Here's the drawing with two shaded views (mm, measured from the low corner). I have some questions. A direction names the side the tool comes from. Give positions to 0.01 mm unless a question says otherwise; leave off trailing zeros. Order: outer loops, then holes, each group sorted by start corner. A loop starts at its lowest first (then second) coordinate and runs counter-clockwise, first axis right, second up. Notation, with made-up numbers: M 6.5,46.25 L 46.5,46.25 A28 cw 46.5,72.25 Z; hole C -6,-3 d7. An arc over 180 degrees is marked long. Use a Markdown table: item, result. Add a question column.
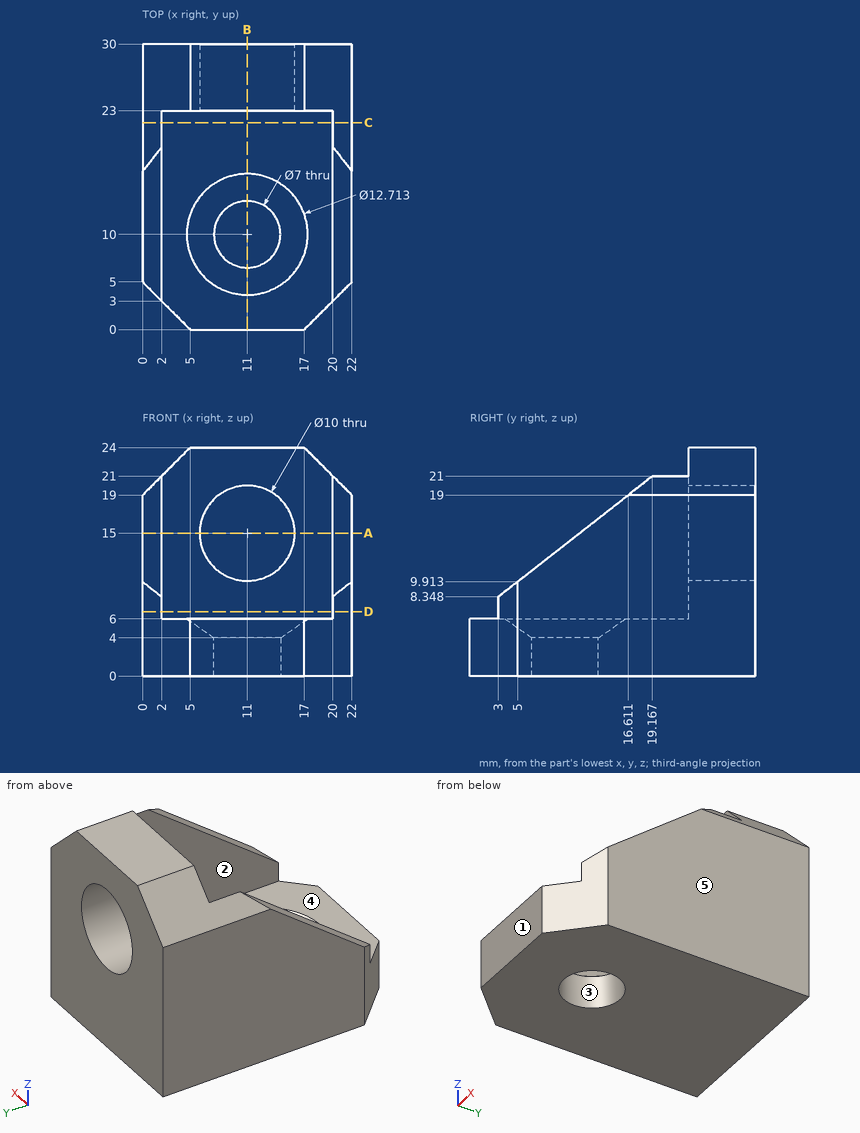
1. If we section it at A-A, the plane z = 15: List the corners of the cut face in (x, y) for me.
2. On a 3-axis mill with a long thin cutter (end or side, diameter ignored), from which of +Z, -Z, +X, -X, +Y, -Y can I reach the whole of each face in a straight line? I mean the marked faces 4 and 5. Say none if no direction works.
3. I need wall thicknesses on L1, parallel to X at y = 13.75, z = 14.25; L2, parallel to Y at x = 11, z = 1.2; L3, parallel to Z at x = 11, y = 28.25. Which ranges of each line are inside material? Lowest first, please. Write a range as [from, to].
4. If we section it at C-C, the plane y = 21.75: List the corners of the cut face in (x, z) for me, then the cut area to 3 significant figures.
5. If we section it at D-D, the plane z = 6.75: List the corners of the cut face in (x, y) for me, then the cut area to 3 significant figures.
6. Will these pins go through, and if not, where does the flat tip stop? pin 1 (9 mm diameter, centred on x = 10.5, z = 18.5, fed in from -Y); pin 2 (10 mm diameter, centred on x = 6.5, y = 8.5, fed in from +Z); pin 3 (9 mm diameter, centred on x = 11, z = 15, fed in from +Y); pin 4 (1.5 mm diameter, centred on y = 3.5, z = 7, fed in from -X).
7. If we section it at B-B, the plane x = 11: List the corners of the cut face in (y, z) for me, then the cut area to 3 significant figures.
8. We'd pull the mould along Y, two halves only. Please class the marked faces 1, 2 and 3: +Y half, -Y half, draft (parallel to the pull), parting line (faces both ways), or undercut.
Geometry results:
| question | item | result |
|---|---|---|
| 1 | outline | M 0,11.5 L 2,11.5 L 2,23 L 6,23 L 6,30 L 0,30 Z; M 16,23 L 20,23 L 20,11.5 L 22,11.5 L 22,30 L 16,30 Z |
| 2 | face 4 | +Z, -Y |
| 2 | face 5 | +Z, -Z, +X, +Y, -Y |
| 3 | L1 | x = [0, 2], [20, 22] |
| 3 | L2 | y = [0, 6.5], [13.5, 30] |
| 3 | L3 | z = [0, 10], [20, 24] |
| 4 | outline | M 0,0 L 22,0 L 22,19 L 20,21 L 20,6 L 2,6 L 2,21 L 0,19 Z |
| 4 | area | 188 mm^2 |
| 5 | outline | M 0,5 L 2,3 L 2,23 L 20,23 L 20,3 L 22,5 L 22,30 L 0,30 Z |
| 5 | area | 230 mm^2 |
| 6 | pin 1 | stops at y = 23 |
| 6 | pin 2 | stops at z = 14.36 |
| 6 | pin 3 | passes through |
| 6 | pin 4 | stops at x = 0.75 |
| 7 | outline | M 0,0 L 6.5,0 L 6.5,4 L 3.64,6 L 0,6 Z; M 13.5,0 L 30,0 L 30,10 L 23,10 L 23,6 L 16.36,6 L 13.5,4 Z; M 23,20 L 30,20 L 30,24 L 23,24 Z |
| 7 | area | 188 mm^2 |
| 8 | face 1 | -Y half |
| 8 | face 2 | draft |
| 8 | face 3 | undercut |
